from build123d import *

# Parameters (mm, degrees)
BOSS_EXTRUDE1_DEPTH     = 25
CUT_EXTRUDE1_DEPTH      = 55.155447556
CUT_EXTRUDE1_DEPTH_BACK = 55.155447556
SKETCH2_R               = 5


with BuildPart() as part:
    # Sketch1 → Boss-Extrude1 (new, symmetric)
    with BuildSketch(Plane(origin=(0, 0, 0), x_dir=(1, 0, 0), z_dir=(0, 1, 0))):
        with BuildLine():
            Line((-43.084219849, 30), (-40, 30))
            ThreePointArc((-40, 30), (0, 50), (40, 30))
            Line((40, 30), (43.084219849, 30))
            ThreePointArc((43.084219849, 30), (0, 52.5), (-43.084219849, 30))
        make_face()
    extrude(amount=BOSS_EXTRUDE1_DEPTH, both=True)

    # Sketch2 → Cut-Extrude1 (cut, two sides: drawn at the far end of the back side and taken through both)
    with BuildSketch(Plane.XY.offset(-51.25).offset(-CUT_EXTRUDE1_DEPTH_BACK)):
        Circle(SKETCH2_R)
    extrude(amount=CUT_EXTRUDE1_DEPTH + CUT_EXTRUDE1_DEPTH_BACK, mode=Mode.SUBTRACT)


solid = part.part
Input: part model. Units: mm. Frame: model coordinates. Give positions to 0.01 mm unless a question says otherwise; leave off trailing zeros. Order: outer loops, then holes, each group sorted by start corner. A loop starts at its lowest first (then second) coordinate and runs counter-clockwise, first axis right, second up. Notation, with made-up numbers: M 64.5,26 L 105.5,26 A23 cw 105.5,58 Z; hole C 64,-1.5 d6. An arc over 180 degrees is marked long. Answer as a JSON object with one key per item and string values.
1. Cut plane B-B, the plane z = -37. Output: boundary loops of the cut face in (x, y).
Result sheet:
{"outline": "M -37.25,-25 L -33.63,-25 L -33.63,25 L -37.25,25 Z; M 33.63,-25 L 37.25,-25 L 37.25,25 L 33.63,25 Z"}
2. Cut plane A-A, the plane x = 0. Output: boundary loops of the cut face in (y, z), and give its area (4 significant figures).
Result sheet:
{"outline": "M -25,-52.5 L -5,-52.5 L -5,-50 L -25,-50 Z; M 5,-52.5 L 25,-52.5 L 25,-50 L 5,-50 Z", "area": "100.0 mm²"}
3. Pull-direction query (X, two-part tool) for faces 1 (the cylindrical face through (-4, 3, -51)), 2 (the cylindrical face through (0.707, 5.906, -52.495)), 3 (the flat face through (-0.2, 25, -50.5)); classes: +X half, -X half, draft (parallel to the pull), parting line (faces both ways), or undercut.
Result sheet:
{"face 1": "undercut", "face 2": "parting line", "face 3": "draft"}
4. Ray query, line 1 (Y direction, x = 0, z = -51.4); line 2 (X direction, y = -9, z = -40); line 3 (X direction, y = -13, z = -44.25). Return the intervals inside material, ascending. Write a range as [from, to].
Result sheet:
{"line 1": "[-25, -5], [5, 25]", "line 2": "[-34, -30], [30, 34]", "line 3": "[-28.25, -23.28], [23.28, 28.25]"}
5. Cut plane D-D, the plane x = -22. Output: boundary loops of the cut face in (y, z).
Result sheet:
{"outline": "M -25,-47.67 L 25,-47.67 L 25,-44.9 L -25,-44.9 Z"}
6. First-contact query: P1, Ø2, axis at x = 17, z = -45.5, coming from the +Y side; P2, Ø5, axis at x = 19, y = 17.5, coming from the -Z side; P3, Ø11.5, axis at x = 0, y = 0, coming from the +Z side; P4, Ø4, axis at x = -28.5, y = -8, coming from the +Z side. Flat tips, straight axial feed; report the tip coordinate or a pass-through.
Result sheet:
{"P1": "through", "P2": "z = -49.84", "P3": "z = -49.67", "P4": "z = -39.62"}
7. Cut plane C-C, the plane y = 7. Output: boundary loops of the cut face in (x, z).
Result sheet:
{"outline": "M -43.08,-30 A52.5 ccw 43.08,-30 L 40,-30 A50 cw -40,-30 Z"}
